Read the model definition and answer for the solid it produces. Units are mm, in the model's axes. Coordinates: 2 decimals unless noted, no trailing zeros. Order: outer loops, then holes, each group sorted by start corner. A loop starts at its lowest first (then second) coordinate and runs counter-clockwise, first axis right, second up. Notation, with made-up numbers: (7, 12.5) -> (11, 12.5) arc R24 ccw to (11, 22.5) -> close; hole circle Ø10 at (-5, 4). An arc over 180 degrees is marked (long way). Return JSON: item names as keys, results as strings. Group by question number.
```python
from build123d import *

# Parameters (mm, degrees)
SKETCH2_R      = 8.336997649
EXTRUDE1_DEPTH = 5.5212


with BuildPart() as part:
    # Sketch1 → Revolve1 (revolve)
    with BuildSketch(Plane.XY):
        Polygon((-1.4478, 0), (-4.4196, 0), (-4.4196, 2.897645717), (-3.482240498, 4.5212), (-1.4478, 4.5212), align=None)
    revolve(axis=Axis((0, 4.5212, 0), (0, -1, 0)))

    # Sketch2 → Extrude1 (cut, through all)
    with BuildSketch(Plane(origin=(0, 0, 0), x_dir=(1, 0, 0), z_dir=(0, 1, 0))):
        Circle(SKETCH2_R)
        Polygon((0, 4.531391323), (-3.9243, 2.265695661), (-3.9243, -2.265695661), (0, -4.531391323), (3.9243, -2.265695661), (3.9243, 2.265695661), align=None, mode=Mode.SUBTRACT)
    extrude(amount=EXTRUDE1_DEPTH, mode=Mode.SUBTRACT)


solid = part.part
```
1. Given pin 1 (1 mm diameter, centred on x = -2.5, y = 1.5, fed in from +Z); pin 2 (2.5 mm diameter, centred on x = 0, z = 0, fed in from -Y), each flat-ended and moving along its own axis, determine where each tip first touches the part or whether it passes through.
2. Find section A-A on z = 0. Determine the outline of the cut face in (x, y).
3. Find section B-B on x = 0. Determine the outline of the cut face in (y, z).
4. Find section D-D on y = 4. Determine the outline of the cut face in (x, z), and give its area (3 significant figures).
5. For a pull along X with two mould halves and no side action, classify faces 1 (the face through (-1.94, 1.85, -3.41)), 2 (the face through (0.314, 2.229, 1.413)), 3 (the face through (1.94, 1.85, 3.41)), 4 (the face through (-0.7, 4.521, 1.5)) as released by +X, released by -X, zero draft, split by the parting line, or undercut.
6. Find section C-C on y = 2.7. Determine the outline of the cut face in (x, z) (3 decimals).
7. Straight lines are drawn through the part: L1, parallel to X at y = 3.05, z = 0; L2, parallel to Y at x = 3.75, z = -0.75; L3, parallel to Z at x = 1.25, y = 1.8. For each, find the intervals that lie inside material, in ascending order.
Result:
{
 "1": {"pin 1": "z = 3.38", "pin 2": "through"},
 "2": {"outline": "(-3.92, 0) -> (-1.45, 0) -> (-1.45, 4.52) -> (-3.48, 4.52) -> (-3.92, 3.76) -> close; (1.45, 0) -> (3.92, 0) -> (3.92, 3.76) -> (3.48, 4.52) -> (1.45, 4.52) -> close"},
 "3": {"outline": "(0, -4.42) -> (2.9, -4.42) -> (4.52, -3.48) -> (4.52, -1.45) -> (0, -1.45) -> close; (0, 1.45) -> (4.52, 1.45) -> (4.52, 3.48) -> (2.9, 4.42) -> (0, 4.42) -> close"},
 "4": {"outline": "circle Ø7.57 at (0, 0); hole circle Ø2.9 at (0, 0)", "area": "38.4 mm^2"},
 "5": {"face 1": "released by -X", "face 2": "undercut", "face 3": "released by +X", "face 4": "zero draft"},
 "6": {"outline": "(-3.924, -2.033) arc R4.42 ccw to (-3.723, -2.382) -> (-0.202, -4.415) arc R4.42 ccw to (0.202, -4.415) -> (3.723, -2.382) arc R4.42 ccw to (3.924, -2.033) -> (3.924, 2.033) arc R4.42 ccw to (3.723, 2.382) -> (0.202, 4.415) arc R4.42 ccw to (-0.202, 4.415) -> (-3.723, 2.382) arc R4.42 ccw to (-3.924, 2.033) -> close; hole circle Ø2.896 at (0, 0)"},
 "7": {"L1": "-3.92 to -1.45, 1.45 to 3.92", "L2": "0 to 3.93", "L3": "-3.81 to -0.73, 0.73 to 3.81"}
}
